Can you work these out from the model? Positions are in its coordinate system, mm. A direction names the side the tool comes from. Give positions to 0.01 mm unless a question says otherwise; leave off trailing zeros. Loops run counter-clockwise (first coordinate to the right, second up) from the corner with the lowest first, then second, coordinate; pieces in that order, holes last. Notation, with made-up numbers: (-11.75, 2) - (44.25, 2) arc R29 cw to (44.25, 27) - close; hole circle Ø9 at (36.5, 82). An arc over 180 degrees is marked (long way). Answer as a JSON object with one key per item and string values.
```python
from build123d import *

# Parameters (mm, degrees)
SKETCH1_W           = 101.6
SKETCH1_H           = 63.5
BOSS_EXTRUDE1_DEPTH = 3.175
SKETCH2_W           = 88.9
SKETCH2_H           = 25.4
CUT_EXTRUDE1_DEPTH  = 4.175
SKETCH3_W           = 3.175
SKETCH3_H           = 12.7
BOSS_EXTRUDE2_DEPTH = 3.175
SKETCH4_W           = 101.6
SKETCH4_H           = 3.175
CUT_EXTRUDE2_DEPTH  = 4.175
CUT_EXTRUDE5_DEPTH  = 4.175


with BuildPart() as part:
    # Sketch1 → Boss-Extrude1 (new body)
    with BuildSketch(Plane.XY):
        with Locations((50.8, 31.75)):
            Rectangle(SKETCH1_W, SKETCH1_H)
    extrude(amount=BOSS_EXTRUDE1_DEPTH)

    # Sketch2 → Cut-Extrude1 (cut, through all)
    with BuildSketch(Plane.XY.offset(3.175)):
        with Locations((50.8, 34.29)):
            Rectangle(SKETCH2_W, SKETCH2_H)
    extrude(amount=-CUT_EXTRUDE1_DEPTH, mode=Mode.SUBTRACT)

    # Sketch3 → Boss-Extrude2 (add)
    with BuildSketch(Plane.XY.offset(3.175)):
        with Locations((-1.5875, 31.75)):
            Rectangle(SKETCH3_W, SKETCH3_H)
        with Locations((103.1875, 31.75)):
            Rectangle(SKETCH3_W, SKETCH3_H)
    extrude(amount=-BOSS_EXTRUDE2_DEPTH)

    # Sketch4 → Cut-Extrude2 (cut, through all)
    with BuildSketch(Plane.XY.offset(3.175)):
        with Locations((50.8, 61.9125)):
            Rectangle(SKETCH4_W, SKETCH4_H)
    extrude(amount=-CUT_EXTRUDE2_DEPTH, mode=Mode.SUBTRACT)

    # Sketch7 → Cut-Extrude5 (cut, through all)
    with BuildSketch(Plane.XY.offset(3.175)):
        with BuildLine():
            Line((6.35, 0), (19.05, 0))
            ThreePointArc((19.05, 0), (12.7, 6.35), (6.35, 0))
        make_face()
        with BuildLine():
            Line((95.25, 0), (82.55, 0))
            ThreePointArc((82.55, 0), (88.9, 6.35), (95.25, 0))
        make_face()
        with BuildLine():
            Line((6.35, 60.325), (19.05, 60.325))
            ThreePointArc((19.05, 60.325), (12.7, 53.975), (6.35, 60.325))
        make_face()
        with BuildLine():
            Line((95.25, 60.325), (82.55, 60.325))
            ThreePointArc((82.55, 60.325), (88.9, 53.975), (95.25, 60.325))
        make_face()
    extrude(amount=-CUT_EXTRUDE5_DEPTH, mode=Mode.SUBTRACT)


solid = part.part
```
1) Imagine slicing it at B-B on z = 2.05. Write out the boundary of the cut face in (x, y) (3 decimals), and give its area (3 significant figures).
Check sheet entries:
{"outline": "(-3.175, 25.4) - (0, 25.4) - (0, 0) - (6.35, 0) arc R6.35 cw to (19.05, 0) - (82.55, 0) arc R6.35 cw to (95.25, 0) - (101.6, 0) - (101.6, 25.4) - (104.775, 25.4) - (104.775, 38.1) - (101.6, 38.1) - (101.6, 60.325) - (95.25, 60.325) arc R6.35 cw to (82.55, 60.325) - (19.05, 60.325) arc R6.35 cw to (6.35, 60.325) - (0, 60.325) - (0, 38.1) - (-3.175, 38.1) - close; hole (6.35, 21.59) - (95.25, 21.59) - (95.25, 46.99) - (6.35, 46.99) - close", "area": "3,700 mm2"}
2) If we mould it in two halves opening along X, with no side actions, what happens to faces 1 (the flat face through (95.25, 34, 2)), 2 (the flat face through (-3.175, 32, 2)), 3 (the flat face through (-2, 25.4, 2)), 4 (the flat face through (104.775, 32, 2))? For each: released by +X, released by -X, zero draft, split by the parting line, or undercut.
Check sheet entries:
{"face 1": "undercut", "face 2": "released by -X", "face 3": "zero draft", "face 4": "released by +X"}
3) I'm going to push flat-ended pins straight in: P1, Ø1, axis at y = 40, z = 1, coming from the -X side; P2, Ø1.6, axis at y = 15, z = 1, coming from the +X side; P3, Ø1, axis at x = -1.5, z = 1.5, coming from the -Y side. Where does each tip first touch, or does it pass through?
Check sheet entries:
{"P1": "x = 0", "P2": "x = 101.6", "P3": "y = 25.4"}
4) Imagine slicing it at A-A on x = 12.7. Write out the boundary of the cut face in (y, z) (3 decimals), and give its area (3 significant figures).
Check sheet entries:
{"outline": "(6.35, 0) - (21.59, 0) - (21.59, 3.175) - (6.35, 3.175) - close; (46.99, 0) - (53.975, 0) - (53.975, 3.175) - (46.99, 3.175) - close", "area": "70.6 mm2"}
5) Which directions (+Z, -Z, +X, -X, +Y, -Y) give clear straight access to the entire face, cutting with the end or side of a thin tool? Please do faces 5 (the flat face through (101.6, 13, 2)), 6 (the flat face through (101.6, 49, 2)), 7 (the flat face through (0, 49, 2)), 8 (the flat face through (50, 46.99, 2)).
Check sheet entries:
{"face 5": "+Z, -Z, +X, -Y", "face 6": "+Z, -Z, +X, +Y", "face 7": "+Z, -Z, -X, +Y", "face 8": "+Z, -Z"}
6) I need wall thicknesses on L1, parallel to X at y = 34.5, z = 2.75 (3 decimals); L2, parallel to Y at x = 29, z = 2.5 (3 decimals); L3, parallel to X at y = 22.5, z = 2.7. Which ranges of each line are inside material? Lowest first, please.
Check sheet entries:
{"L1": "-3.175 to 6.35, 95.25 to 104.775", "L2": "0 to 21.59, 46.99 to 60.325", "L3": "0 to 6.35, 95.25 to 101.6"}
7) Imagine slicing it at C-C on x = 42.5. Write out the boundary of the cut face in (y, z) (3 decimals).
Check sheet entries:
{"outline": "(0, 0) - (21.59, 0) - (21.59, 3.175) - (0, 3.175) - close; (46.99, 0) - (60.325, 0) - (60.325, 3.175) - (46.99, 3.175) - close"}
8) Imagine slicing it at D-D on y = 12.5. Write out the boundary of the cut face in (x, z) (3 decimals).
Check sheet entries:
{"outline": "(0, 0) - (101.6, 0) - (101.6, 3.175) - (0, 3.175) - close"}
